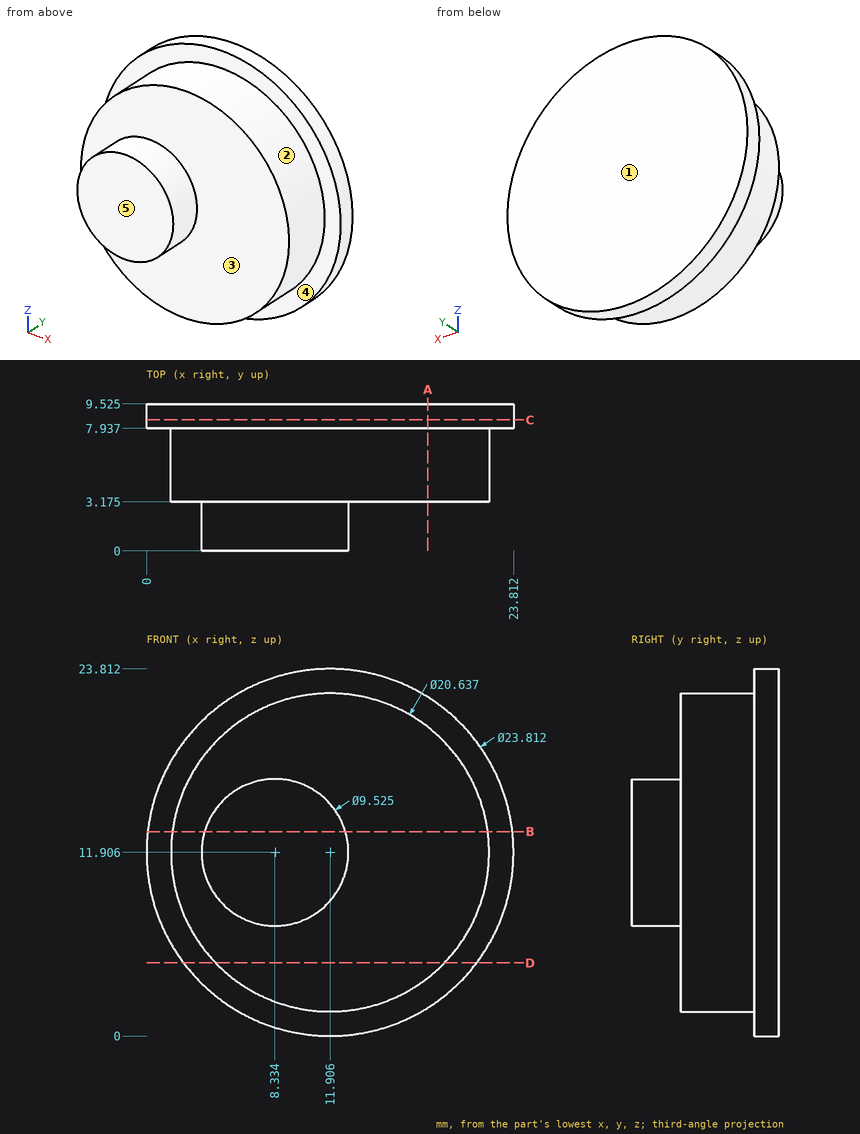
Study the drawing (mm; zero at the part's minimum x, y, z) and answer. A direction names the side the tool comes from. Give positions to 0.01 mm unless a question says otherwise; leave off trailing zeros. Write each loop counter-clockwise with the first axis right and the second up, starting at its lowest first coordinate (ties: lowest second). Pieces come first, ordered by that corner, then holes. Notation, with made-up numbers: (-38.75, -20) -> (-26.75, -20) arc R16 ccw to (-26.75, -6) -> close; hole circle Ø6 at (20.25, 77.5). An arc over 180 degrees is marked (long way). Answer as a JSON object with one key per item and string values. Group by question number.
1) A tool of negligible diameter and unlimited length cuts with its end or side. For the marked faces 4 and 5, from which of +Z, -Z, +X, -X, +Y, -Y can it reach the whole face along a straight path? Write none if from no direction.
2) Find section C-C (y = 8.5). Write down the section's boundary in (x, z), and give its area (3 significant figures).
3) Find section D-D (z = 4.75). Write down the section's boundary in (x, y) (1 decimal).
4) Each of these flat-tipped pins is pushed along its axis until it touches: P1, Ø1.5, axis at x = 11.5, y = 5.5, coming from the -Z side; P2, Ø3, axis at x = 3, y = 2, coming from the +Z side (1 decimal); P3, Ø3, axis at x = 7.5, y = 6, coming from the -Z side (1 decimal). Where does it stop, or does it pass through?
5) The mould has two halves that part along Y. Classify the marked faces 1, 2 and 3: +Y half, -Y half, draft (parallel to the pull), parting line (faces both ways), or undercut.
6) Find section A-A (x = 18.25). Write down the section's boundary in (y, z) (1 decimal).
7) Consider L1, parallel to Y at x = 18, z = 8 (1 decimal); L2, parallel to X at y = 6, z = 5 (1 decimal); L3, parallel to X at y = 8.5, z = 3.5 (1 decimal). Determine where each line is inside the solid, lowest interval first. Write a range as from..to.
8) Find section B-B (z = 13.25). Write down the section's boundary in (x, y) (1 decimal), and give its area (3 significant figures).
Values follow:
{
 "1": {"face 4": "-Y", "face 5": "+Z, -Z, +X, -X, -Y"},
 "2": {"outline": "circle Ø23.81 at (11.91, 11.91)", "area": "445 mm2"},
 "3": {"outline": "(2.4, 7.9) -> (4.5, 7.9) -> (4.5, 3.2) -> (19.3, 3.2) -> (19.3, 7.9) -> (21.4, 7.9) -> (21.4, 9.5) -> (2.4, 9.5) -> close"},
 "4": {"P1": "stops at z = 1.59", "P2": "stops at z = 18.5", "P3": "stops at z = 2"},
 "5": {"face 1": "+Y half", "face 2": "draft", "face 3": "-Y half"},
 "6": {"outline": "(3.2, 3.8) -> (7.9, 3.8) -> (7.9, 1.8) -> (9.5, 1.8) -> (9.5, 22) -> (7.9, 22) -> (7.9, 20) -> (3.2, 20) -> close"},
 "7": {"L1": "y = 3.2..9.5", "L2": "x = 4.2..19.6", "L3": "x = 3.5..20.3"},
 "8": {"outline": "(0.1, 7.9) -> (1.7, 7.9) -> (1.7, 3.2) -> (3.8, 3.2) -> (3.8, 0) -> (12.9, 0) -> (12.9, 3.2) -> (22.1, 3.2) -> (22.1, 7.9) -> (23.7, 7.9) -> (23.7, 9.5) -> (0.1, 9.5) -> close", "area": "164 mm2"}
}
